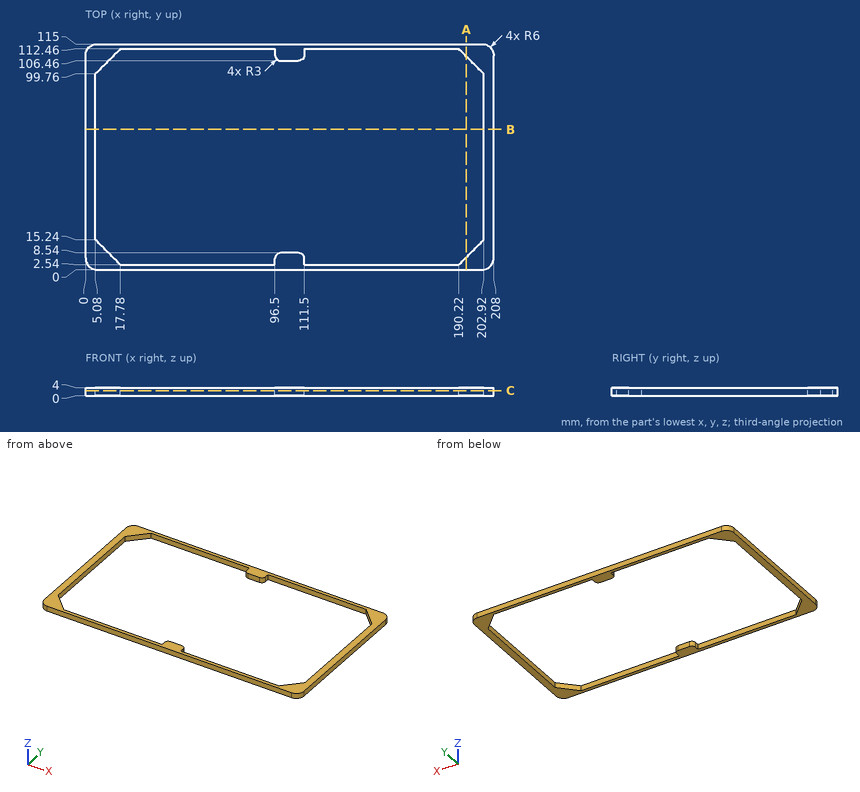
Job drawing, mm, ordinate dimensions from the low corner. One solid piece. Coordinates: 2 decimals unless noted, no trailing zeros. Order: outer loops, then holes, each group sorted by start corner. A loop starts at its lowest first (then second) coordinate and runs counter-clockwise, first axis right, second up. Notation, with made-up numbers: (5.5, -29) - (48.5, -29) arc R17 cw to (48.5, 3) - close; hole circle Ø8 at (77.5, 72). An arc over 180 degrees is marked (long way). Return JSON: item names as keys, results as strings. Group by question number.
1) Saw through at C-C, the plane z = 2.5. Write the cut outline in (x, y).
2) Saw through at B-B, the plane y = 71.5. Write the cut outline in (x, z).
3) Saw through at A-A, the plane x = 194. Write the cut outline in (y, z), plus the area to 3 significant figures.
4) Probe line 1 (X direction, y = 35, z = 0.3); line 2 (Y direction, x = 171.5, z = 2.9); line 3 (Y direction, x = 107.5, z = 0.4). List the from-to ranges inside material, lowest first. Write a range as from..to.
5) Flat gauge pins, fed straight in: P1, Ø0.9, axis at y = 110, z = 1.5, coming from the -X side; P2, Ø0.9, axis at y = 111, z = 2, coming from the +X side. Where does each tip first touch, or does it go through?
Values found:
{
 "1": {"outline": "(0, 6) arc R6 ccw to (6, 0) - (202, 0) arc R6 ccw to (208, 6) - (208, 109) arc R6 ccw to (202, 115) - (6, 115) arc R6 ccw to (0, 109) - close; hole (5.08, 15.24) - (17.78, 2.54) - (96.5, 2.54) - (96.5, 5.54) arc R3 cw to (99.5, 8.54) - (108.5, 8.54) arc R3 cw to (111.5, 5.54) - (111.5, 2.54) - (190.22, 2.54) - (202.92, 15.24) - (202.92, 99.76) - (190.22, 112.46) - (111.5, 112.46) - (111.5, 109.46) arc R3 cw to (108.5, 106.46) - (99.5, 106.46) arc R3 cw to (96.5, 109.46) - (96.5, 112.46) - (17.78, 112.46) - (5.08, 99.76) - close"},
 "2": {"outline": "(0, 0) - (5.08, 0) - (5.08, 4) - (0, 4) - close; (202.92, 0) - (208, 0) - (208, 4) - (202.92, 4) - close"},
 "3": {"outline": "(0, 0) - (6.32, 0) - (6.32, 4) - (0, 4) - close; (108.68, 0) - (115, 0) - (115, 4) - (108.68, 4) - close", "area": "50.6 mm²"},
 "4": {"line 1": "x = 0..5.08, 202.92..208", "line 2": "y = 0..2.54, 112.46..115", "line 3": "y = 0..8.54, 106.46..115"},
 "5": {"P1": "stops at x = 0.03", "P2": "stops at x = 207.8"}
}
